Read the model definition and answer for the solid it produces. Units are mm, in the model's axes. Give positions to 0.01 mm unless a question says otherwise; leave off trailing zeros. Order: outer loops, then holes, each group sorted by start corner. A loop starts at its lowest first (then second) coordinate and runs counter-clockwise, first axis right, second up.
```python
from build123d import *

# Parameters (mm, degrees)
F0_R     = 3
F0_R_2   = 2
F1_DEPTH = 5
F0_R_3   = 4
F2_DEPTH = 5
F3_DEPTH = 3


with BuildPart() as f1:
    # F0 (on Front) → F1 (new body)
    with BuildSketch(Plane.XZ):
        Circle(F0_R)
        Circle(F0_R_2, mode=Mode.SUBTRACT)
    extrude(amount=-F1_DEPTH)

    # F0 (on Front) → F2 (join)
    with BuildSketch(Plane.XZ):
        Circle(F0_R_3)
        Circle(F0_R, mode=Mode.SUBTRACT)
    extrude(amount=-F2_DEPTH)

    # F0 (on Front) → F3 (join)
    with BuildSketch(Plane.XZ):
        Circle(F0_R)
        Circle(F0_R_2, mode=Mode.SUBTRACT)
    extrude(amount=F3_DEPTH)


solid = f1.part
```
1) For a pull along Z with two mould halves and no side action, classify faces 1 (the face through (1, 0, 3)), 2 (the face through (-3, -1, 0)), 3 (the face through (0, 1, -2)) as released by +Z, released by -Z, zero draft, split by the parting line, or undercut.
Final values:
face 1: zero draft
face 2: split by the parting line
face 3: undercut
2) Consider L1, parallel to Z at x = 0, y = 2.25; L2, parallel to Y at x = 3, z = -0.5; L3, parallel to Z at x = -1, y = -1.25. Determine where each line is inside the solid, lowest interval first.
Final values:
L1: z = -4 to -2, 2 to 4
L2: y = 0 to 5
L3: z = -2.83 to -1.73, 1.73 to 2.83
3) The part is cut by section D-D on y = -1. Determine the outline of the cut face in (x, z), and give its area (3 significant figures).
Final values:
outline: circle Ø6 at (0, 0); hole circle Ø4 at (0, 0)
area: 15.7 mm2
4) Given pin 1 (2.5 mm diameter, centred on x = 0, z = 0, fed in from +Y); pin 2 (4 mm diameter, centred on x = 1, z = -0.5, fed in from -Y); pin 3 (2 mm diameter, centred on y = -2, z = -1, fed in from +X), each flat-ended and moving along its own axis, determine where each tip first touches the part or whether it passes through.
Final values:
pin 1: passes through
pin 2: stops at y = -3
pin 3: stops at x = 3
5) The part is cut by section C-C on y = 4. Determine the outline of the cut face in (x, z), and give its area (3 significant figures).
Final values:
outline: circle Ø8 at (0, 0); hole circle Ø4 at (0, 0)
area: 37.7 mm2
6) The part is cut by section B-B on x = 0. Determine the outline of the cut face in (y, z), and give its area (3 significant figures).
Final values:
outline: (-3, -3) - (0, -3) - (0, -4) - (5, -4) - (5, -2) - (-3, -2) - close; (-3, 2) - (5, 2) - (5, 4) - (0, 4) - (0, 3) - (-3, 3) - close
area: 26.0 mm2
7) The part is cut by section A-A on z = -0.25. Determine the outline of the cut face in (x, y).
Final values:
outline: (-3.99, 0) - (-2.99, 0) - (-2.99, -3) - (-1.98, -3) - (-1.98, 5) - (-3.99, 5) - close; (1.98, -3) - (2.99, -3) - (2.99, 0) - (3.99, 0) - (3.99, 5) - (1.98, 5) - close
